```python
from build123d import *

# Parameters (mm, degrees)
SKETCH001_R      = 9
EXTRUDE001_DEPTH = 5
SKETCH002_R      = 9.5
EXTRUDE002_DEPTH = 4
SKETCH003_R      = 11
EXTRUDE003_DEPTH = 3.5
SKETCH004_R      = 12
EXTRUDE004_DEPTH = 2.5
SKETCH_R         = 7.5
EXTRUDE_DEPTH    = 6


with BuildPart() as extrude001:
    # Sketch001 → Extrude001 (new body)
    with BuildSketch(Plane.XY):
        Circle(SKETCH001_R)
    extrude(amount=EXTRUDE001_DEPTH)


with BuildPart() as extrude002:
    # Sketch002 → Extrude002 (new body)
    with BuildSketch(Plane.XY):
        Circle(SKETCH002_R)
    extrude(amount=EXTRUDE002_DEPTH)


with BuildPart() as extrude003:
    # Sketch003 → Extrude003 (new body)
    with BuildSketch(Plane.XY):
        Circle(SKETCH003_R)
    extrude(amount=EXTRUDE003_DEPTH)


with BuildPart() as extrude004:
    # Sketch004 → Extrude004 (new body)
    with BuildSketch(Plane.XY):
        Circle(SKETCH004_R)
    extrude(amount=EXTRUDE004_DEPTH)


with BuildPart() as fusion:
    # Sketch → Extrude (new body)
    with BuildSketch(Plane.XY):
        Circle(SKETCH_R)
    extrude(amount=EXTRUDE_DEPTH)

    # Fusion: union Extrude001, Extrude002, Extrude003, Extrude004
    add(extrude001.part)
    add(extrude002.part)
    add(extrude003.part)
    add(extrude004.part)


solid = fusion.part
```
Could you check a few things on this model? Use its own coordinates, in mm. A direction names the side the tool comes from. Round coordinates to 2 decimals unless told otherwise and drop trailing zeros. Loops run counter-clockwise (first coordinate to the right, second up) from the corner with the lowest first, then second, coordinate; pieces in that order, holes last. Notation, with made-up numbers: M 1,11 L 54,11 A28 ccw 54,31 Z; hole C -34,54 d1. An arc over 180 degrees is marked long. Answer as CSV lines item,"result".
1) If I drill on probe 1 along Z at (x, y) = (1.25, 10.75); probe 2 along Z at (x, y) = (5, -5.75); probe 3 along Y at (x, z) = (2, 0.45), over which ranges is the centre line in solid material (lowest first)?
From the geometry:
probe 1,"0 to 3.5"
probe 2,"0 to 5"
probe 3,"-11.83 to 11.83"
2) For pin 1 Ø1.5 at (x, z) = (-4.5, 1) entering from +Y; pin 2 Ø2 at (x, y) = (8, -4) entering from +Z; pin 3 Ø3 at (y, z) = (-3, 2) entering from -X, each with a flat end and sliding along its axis, tell me the tip position at first contact or that it passes through.
From the geometry:
pin 1,"y = 11.4"
pin 2,"z = 5"
pin 3,"x = -11.91"
3) Imagine slicing it at C-C on z = 5.35. List the corners of the cut face in (x, y) for me, and give its area (3 significant figures).
From the geometry:
outline,"C 0,0 d15"
area,"177 mm^2"
4) Imagine slicing it at D-D on z = 1.75. List the corners of the cut face in (x, y) for me, and give its area (3 significant figures).
From the geometry:
outline,"C 0,0 d24"
area,"452 mm^2"
5) Imagine slicing it at A-A on y = 0. List the corners of the cut face in (x, z) for me.
From the geometry:
outline,"M -12,0 L 12,0 L 12,2.5 L 11,2.5 L 11,3.5 L 9.5,3.5 L 9.5,4 L 9,4 L 9,5 L 7.5,5 L 7.5,6 L -7.5,6 L -7.5,5 L -9,5 L -9,4 L -9.5,4 L -9.5,3.5 L -11,3.5 L -11,2.5 L -12,2.5 Z"
6) Which directions (+Z, -Z, +X, -X, +Y, -Y) give clear straight access to the entire face, cutting with the end or side of a thin tool? Please do faces 1 (the flat face through (0, 0, 0)), 2 (the flat face through (-2, 7.4, 5)).
From the geometry:
face 1,"-Z, +X, -X, +Y, -Y"
face 2,"+Z"
